The listing builds one solid part. Answer for the finished solid, in the listing's coordinates (mm). A direction names the side the tool comes from. Coordinates: 2 decimals unless noted, no trailing zeros. Order: outer loops, then holes, each group sorted by start corner. A loop starts at its lowest first (then second) coordinate and runs counter-clockwise, first axis right, second up. Notation, with made-up numbers: (56.5, 29) - (63.5, 29) arc R26 cw to (63.5, 49) - close; hole circle Ø7 at (63.25, -24). An arc over 180 degrees is marked (long way). Use a Markdown table: item, result. Add a question column.
Item 1: The part is cut by section D-D, the plane x = -87.75. Give the vertices of the cut face in (y, z).
Item 2: Flat-ended cylindrical pins translate along their axes: P1, Ø2.5, axis at x = -90, z = -3.5, coming from the -Y side; P2, Ø4, axis at x = -89, y = 1, coming from the +Z side; P3, Ø2.5, axis at x = -87.5, z = 7, coming from the +Y side; P4, Ø1.9, axis at x = -87.93, z = 6.45, coming from the +Y side. Find the tip coordinate at first contact, or state that the pin passes through.
Item 3: For faces 4 (the flat face through (-92.43, -2, 3)), 5 (the flat face through (-88, 0, 0)), 6 (the flat face through (-88, 3, 2)), 7 (the cylindrical face through (-91.23, -2.25, 6.3)), 8 (the flat face through (-88, -5.25, 4)), determine the directions among +Z, -Z, +X, -X, +Y, -Y from which every point of the face is accessible in a straight line to the end or side of a thin tool.
Item 4: The mould has two halves that part along X. Classify faces 1 (the flat face through (-88, 5, -5)), 2 (the flat face through (-83.43, -2, 3)), 3 (the cylindrical face through (-89.397, -4.28, 7.056)): released by +X, released by -X, zero draft, split by the parting line, or undercut.
Item 5: The part is cut by section A-A, the plane x = -86.75. Give the vertices of the cut face in (y, z).
Item 6: The part is cut by section C-C, the plane z = 7.75. Give the vertices of the cut face in (x, y).
Item 7: Find the intervals of material crossed by line 1 along Z through (x, y) = (-87.75, -2.5); line 2 along Y through (x, z) = (-86.75, 9.5); line 3 along X through (y, z) = (-3, 8.25), in increasing order.
Item 8: The part is cut by section B-B, the plane y = -4.25. Give the vertices of the cut face in (x, z) (1 decimal).
from build123d import *

# Parameters (mm, degrees)
SKETCH1_W                                           = 9
SKETCH1_H                                           = 11.7
BOSS_EXTRUDE1_DEPTH                                 = 2
SKETCH2_W                                           = 9
SKETCH2_H                                           = 2
BOSS_EXTRUDE2_DEPTH                                 = 5
SKETCH3_W                                           = 9
SKETCH3_H                                           = 4
BOSS_EXTRUDE3_DEPTH                                 = 9
CBORE_FOR_4_BINDING_HEAD_MACHINE_SCREW1_D           = 3.175
CBORE_FOR_4_BINDING_HEAD_MACHINE_SCREW1_CBORE_D     = 6.604
CBORE_FOR_4_BINDING_HEAD_MACHINE_SCREW1_CBORE_DEPTH = 2.032


with BuildPart() as part:
    # Sketch1 → Boss-Extrude1 (new body)
    with BuildSketch(Plane.XY):
        with Locations((-87.930083344, 0.6)):
            Rectangle(SKETCH1_W, SKETCH1_H)
    extrude(amount=BOSS_EXTRUDE1_DEPTH)

    # Sketch2 → Boss-Extrude2 (add)
    with BuildSketch(Plane(origin=(0, 0, 0), x_dir=(-1, 0, 0), z_dir=(0, 0, -1))):
        with Locations((87.930083344, 5.45)):
            Rectangle(SKETCH2_W, SKETCH2_H)
    extrude(amount=BOSS_EXTRUDE2_DEPTH)

    # Sketch3 → Boss-Extrude3 (add)
    with BuildSketch(Plane.XY.offset(2)):
        with Locations((-87.930083344, -3.25)):
            Rectangle(SKETCH3_W, SKETCH3_H)
    extrude(amount=BOSS_EXTRUDE3_DEPTH)

    # CBORE for #4 Binding Head Machine Screw1 (through all)
    with Locations(Plane(origin=(0, -1.25, 0), x_dir=(1, 0, 0), z_dir=(0, 1, 0))):
        with Locations((-87.930083344, -6.448155288)):
            CounterBoreHole(CBORE_FOR_4_BINDING_HEAD_MACHINE_SCREW1_D / 2, CBORE_FOR_4_BINDING_HEAD_MACHINE_SCREW1_CBORE_D / 2, CBORE_FOR_4_BINDING_HEAD_MACHINE_SCREW1_CBORE_DEPTH)


solid = part.part
Solution:
| question | item | result |
|---|---|---|
| 1 | outline | (-5.25, 0) - (4.45, 0) - (4.45, -5) - (6.45, -5) - (6.45, 2) - (-1.25, 2) - (-1.25, 3.15) - (-3.28, 3.15) - (-3.28, 4.87) - (-5.25, 4.87) - close; (-5.25, 8.03) - (-3.28, 8.03) - (-3.28, 9.75) - (-1.25, 9.75) - (-1.25, 11) - (-5.25, 11) - close |
| 2 | P1 | stops at y = 4.45 |
| 2 | P2 | stops at z = 2 |
| 2 | P3 | stops at y = -3.28 |
| 2 | P4 | passes through |
| 3 | face 4 | +Z, -Z, -X, +Y, -Y |
| 3 | face 5 | -Z, +X, -X, -Y |
| 3 | face 6 | +Z, +X, -X, +Y |
| 3 | face 7 | +Y |
| 3 | face 8 | +Z, -Z, +X, -X, -Y |
| 4 | face 1 | zero draft |
| 4 | face 2 | released by +X |
| 4 | face 3 | undercut |
| 5 | outline | (-5.25, 0) - (4.45, 0) - (4.45, -5) - (6.45, -5) - (6.45, 2) - (-1.25, 2) - (-1.25, 3.36) - (-3.28, 3.36) - (-3.28, 5.39) - (-5.25, 5.39) - close; (-5.25, 7.51) - (-3.28, 7.51) - (-3.28, 9.53) - (-1.25, 9.53) - (-1.25, 11) - (-5.25, 11) - close |
| 6 | outline | (-92.43, -5.25) - (-88.84, -5.25) - (-88.84, -3.28) - (-90.96, -3.28) - (-90.96, -1.25) - (-92.43, -1.25) - close; (-87.02, -5.25) - (-83.43, -5.25) - (-83.43, -1.25) - (-84.9, -1.25) - (-84.9, -3.28) - (-87.02, -3.28) - close |
| 7 | line 1 | z = 0 to 3.15, 9.75 to 11 |
| 7 | line 2 | y = -5.25 to -3.28 |
| 7 | line 3 | x = -92.43 to -90.7, -85.16 to -83.43 |
| 8 | outline | (-92.4, 0) - (-83.4, 0) - (-83.4, 11) - (-92.4, 11) - close; hole circle Ø3.2 at (-87.9, 6.4) |
